```python
from build123d import *

# Parameters (mm, degrees)
F1_DEPTH = 12.7
F2_DEPTH = 6.35


with BuildPart() as f1:
    # F0 (on Top) → F1 (new body)
    with BuildSketch(Plane.XY):
        Polygon((22.474717, 12.095485), (-20.022932, 36.940265), (-41.326346, 50.449748), (-24.396872, 34.043866), (-15.936619, 23.769072), (-31.791512, 23.769072), (-3.187324, 1.866438), (-22.801625, 1.866438), (29.666629, -31.641328), (48.181905, -43.382723), (33.589493, -29.257998), (15.119358, -10.951318), (33.589493, -10.951318), (4.004587, 12.095485), align=None)
    extrude(amount=F1_DEPTH)

    # F0 (on Top) → F2 (join)
    with BuildSketch(Plane.XY):
        Polygon((4.004587, 41.190032), (0, 41.190032), (-8.744708, 39.88241), (-20.022932, 36.940265), (22.474717, 12.095485), (4.004587, 12.095485), (33.589493, -10.951318), (15.119358, -10.951318), (33.589493, -29.257998), (38.892256, -23.779654), (42.238043, -18.503606), (46.43552, -11.884507), (46.43552, -3.675631), (46.43552, 5.557385), (44.213898, 11.76858), (41.435212, 19.123944), (38.166158, 23.700614), (31.46461, 30.72907), (22.434429, 36.455527), (14.13864, 39.718959), align=None)
        Polygon((22.474717, 12.095485), (-20.022932, 36.940265), (-41.326346, 50.449748), (-24.396872, 34.043866), (-15.936619, 23.769072), (-31.791512, 23.769072), (-3.187324, 1.866438), (-22.801625, 1.866438), (29.666629, -31.641328), (48.181905, -43.382723), (33.589493, -29.257998), (15.119358, -10.951318), (33.589493, -10.951318), (4.004587, 12.095485), align=None)
        Polygon((-15.936619, 23.769072), (-24.396872, 34.043866), (-31.791512, 26.413227), (-36.553774, 20.371506), (-40.454496, 14.220368), (-42.415924, 5.557385), (-42.415924, -5.720838), (-40.454496, -14.242595), (-33.426039, -24.517875), (-20.022932, -35.632648), (-6.456373, -40.209316), (4.331491, -40.209316), (17.080786, -37.920982), (25.580317, -34.161571), (29.666629, -31.641328), (-22.801625, 1.866438), (-3.187324, 1.866438), (-31.791512, 23.769072), align=None)
    extrude(amount=F2_DEPTH)


solid = f1.part
```
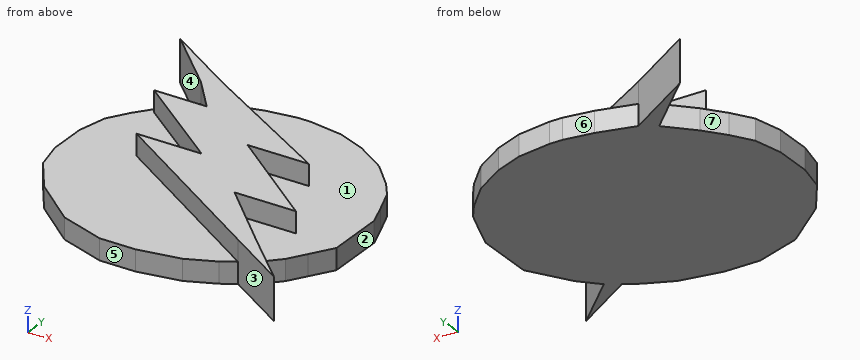
The model under review builds one solid part; all positions refer to its coordinate system, in mm. Face numbers are marked on the shaded views. A direction names the side the tool comes from. Give positions to 0.01 mm unless a question says otherwise; leave off trailing zeros. Write each loop counter-clockwise with the first axis right and the second up, starting at its lowest first coordinate (ties: lowest second). Pieces come first, ordered by that corner, then holes.
(1) To check wall thickness, follow L1, parallel to Z at x = 15, y = -37; L2, parallel to Y at x = 12.5, z = 6.5; L3, parallel to Y at x = -20, z = 11.25. State the ranges of each line that lie inside material, in increasing order.
(2) Consider section C-C, the plane y = 0.5. Give the boundary of the cut face in (x, z), and give its area (3 significant figures).
(3) Consider section D-D, the plane x = 20.5. Give the boundary of the cut face in (y, z).
(4) Tool access review of the marked faces 5, 6 and 7: name each direction out of +Z, -Z, +X, -X, +Y, -Y from which nothing blocks a thin tool from reaching the whole face with its end or side.
(5) Consider section B-B, the plane x = -35. Give the boundary of the cut face in (y, z).
(6) The part is to be moulded in two halves that separate along X. For the marked faces 1, 2, 3 and 4, say which applies: released by +X, released by -X, zero draft, split by the parting line, or undercut.
(7) For P1, Ø1.5, axis at x = -24.5, z = 2, coming from the -Y side; P2, Ø3, axis at x = -21.5, z = 9.5, coming from the +Y side; P3, Ø5, axis at x = 11, z = 9, coming from the -Y side, all flat-tipped, find the tip position at first contact; note any pin that passes through.
(8) Consider section A-A, the plane z = 8. Give the boundary of the cut face in (x, y), and give its area (3 significant figures).
Returned:
1. L1: z = 0 to 6.35
1. L2: y = -20.68 to 5.48, 12.1 to 17.93
1. L3: y = 0.08 to 1.87, 14.74 to 23.77, 28.7 to 36.93
2. outline: (-42.42, 0) - (46.44, 0) - (46.44, 6.35) - (18.89, 6.35) - (18.89, 12.7) - (-20.66, 12.7) - (-20.66, 6.35) - (-42.42, 6.35) - close
2. area: 815 mm2
3. outline: (-36.41, 0) - (37.22, 0) - (37.22, 6.35) - (13.25, 6.35) - (13.25, 12.7) - (12.1, 12.7) - (12.1, 6.35) - (-0.75, 6.35) - (-0.75, 12.7) - (-10.95, 12.7) - (-10.95, 6.35) - (-16.28, 6.35) - (-16.28, 12.7) - (-25.79, 12.7) - (-25.79, 6.35) - (-36.41, 6.35) - close
4. face 5: +Z, -Z, -X, -Y
4. face 6: +Z, -Z, +Y
4. face 7: +Z, -Z, -X
5. outline: (-22.22, 0) - (22.34, 0) - (22.34, 6.35) - (-22.22, 6.35) - close; (44.32, 0) - (46.44, 0) - (46.44, 12.7) - (44.32, 12.7) - close
6. face 1: zero draft
6. face 2: released by +X
6. face 3: undercut
6. face 4: released by -X
7. P1: stops at y = -32.54
7. P2: stops at y = 38.83
7. P3: stops at y = -21.32
8. outline: (-41.33, 50.45) - (-24.4, 34.04) - (-15.94, 23.77) - (-31.79, 23.77) - (-3.19, 1.87) - (-22.8, 1.87) - (29.67, -31.64) - (48.18, -43.38) - (33.59, -29.26) - (15.12, -10.95) - (33.59, -10.95) - (4, 12.1) - (22.47, 12.1) - (-20.02, 36.94) - close
8. area: 1,630 mm2
